Source: CAD feature listing. Evaluate the final solid. Frame: model axes, mm. Face numbers are marked on the shaded views. A direction names the side the tool comes from. Coordinates: 2 decimals unless noted, no trailing zeros. Write each loop counter-clockwise with the first axis right and the second up, starting at its lowest first coordinate (ties: lowest second). Pieces come first, ordered by that corner, then holes. Notation, with made-up numbers: (-39.5, 2) - (-10.5, 2) arc R23 cw to (-10.5, 35) - close; hole circle Ø4 at (19, -13). An arc over 180 degrees is marked (long way). One line per item, written item: value.
Autodesk Inventor part; units mm, degrees
ref_plane "YZ Plane" through (0, 0, 0) normal (1, 0, 0) x (0, 1, 0)
ref_plane "XZ Plane" through (0, 0, 0) normal (0, 1, 0) x (-1, 0, 0)
ref_plane "XY Plane" through (0, 0, 0) normal (0, 0, 1) x (1, 0, 0)
sketch "sketch" plane through (0, 0, 0) normal (0, 0, 1) x (1, 0, 0)
  line L0 (-7.2, 0) -> (43.2, 0) construction
  line L1 (0, -3.36) -> (0, 20.16) construction
  line L2 (3, 13.8) -> (33, 13.8)
  line L3 (33, 13.8) -> (33, 3)
  line L4 (33, 3) -> (3, 3)
  line L5 (3, 3) -> (3, 13.8)
  line L6 (18, 11.9) -> (33, 11.9)
  line L7 (33, 11.9) -> (33, 4.9)
  line L8 (33, 4.9) -> (18, 4.9)
  line L9 (18, 4.9) -> (18, 11.9)
  line L10 (36, 16.8) -> (0, 16.8)
  line L11 (0, 16.8) -> (0, 0)
  line L12 (0, 0) -> (36, 0)
  line L13 (36, 0) -> (36, 16.8)
  line L14 (33, 4.9) -> (36, 4.9)
  line L15 (33, 11.9) -> (36, 11.9)
  line L16 (0, 3) -> (3, 3)
  line L17 (0, 13.8) -> (3, 13.8)
  line L18 (33, 3) -> (36, 3)
  line L19 (33, 13.8) -> (36, 13.8)
  dimension "d0" = 10.8
  dimension "d2" = 7
  dimension "d3" = 1.9
  dimension "d4" = 15
  dimension "d5" = 30
  dimension "d6" = 3
extrude "돌출1" add sketch "sketch" along normal blind 15
extrude "floor" cut sketch "sketch" along normal blind 12 contours L2 L3 L6 L9 L8 L4 L5 | L5 L16 L11 L17 | L19 L13 L15 L3 | L3 L14 L13 L18
extrude "fix" cut sketch "sketch" along normal up to surface (15 mm away) contours L15 L13 L14 L3 | L3 L8 L9 L6
equation "\"d3\" = -0.5 * d2 + 0.5 * d0"
properties part number "button_fix"
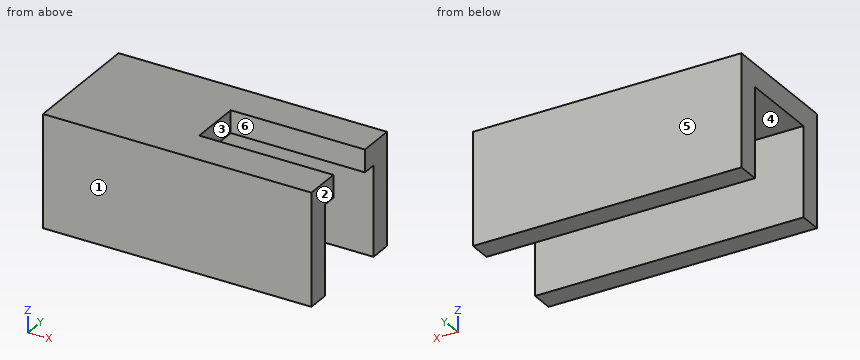
1) Reachability of the marked faces 4, 5 and 6 from +Z, -Z, +X, -X, +Y, -Y: full face, straight path, thin tool, end or side. Return the list, or none.
Values found:
face 4: -Z, +X, -X
face 5: +Z, -Z, +X, -X, +Y
face 6: +Z, -Z, +X
2) Section query D-D on z = 13. Output: boundary loops of the cut face in (x, y).
Values found:
outline: (0, 0) - (36, 0) - (36, 4.9) - (18, 4.9) - (18, 11.9) - (36, 11.9) - (36, 16.8) - (0, 16.8) - close
3) Contact query for flat-ended pins moving along their axis: P1, Ø2.5, axis at y = 9.5, z = 13.5, coming from the +X side; P2, Ø3, axis at x = 26, y = 10.5, coming from the -Z side. Output: stop coordinate, or through.
Values found:
P1: x = 18
P2: z = 12
4) Section query A-A on z = 9. Output: boundary loops of the cut face in (x, y), then the cut area to 3 significant figures.
Values found:
outline: (0, 0) - (36, 0) - (36, 3) - (0, 3) - close; (0, 13.8) - (36, 13.8) - (36, 16.8) - (0, 16.8) - close
area: 216 mm2
5) Material intervals for line 1 (Y direction, x = 10.5, z = 7); line 2 (Y direction, x = 31, z = 12.75); line 3 (X direction, y = 5.5, z = 14.25), sorted ascending.
Values found:
line 1: 0 to 3, 13.8 to 16.8
line 2: 0 to 4.9, 11.9 to 16.8
line 3: 0 to 18
6) Section query C-C on x = 16.5. Output: boundary loops of the cut face in (y, z), then the cut area to 3 significant figures.
Values found:
outline: (0, 0) - (3, 0) - (3, 12) - (13.8, 12) - (13.8, 0) - (16.8, 0) - (16.8, 15) - (0, 15) - close
area: 122 mm2
7) Draft query along Y for the marked faces 1, 2 and 3. Return one class per face: released by +Y, released by -Y, zero draft, split by the parting line, or undercut.
Values found:
face 1: released by -Y
face 2: zero draft
face 3: undercut
8) Section query B-B on x = 26. Output: boundary loops of the cut face in (y, z).
Values found:
outline: (0, 0) - (3, 0) - (3, 12) - (4.9, 12) - (4.9, 15) - (0, 15) - close; (11.9, 12) - (13.8, 12) - (13.8, 0) - (16.8, 0) - (16.8, 15) - (11.9, 15) - close
